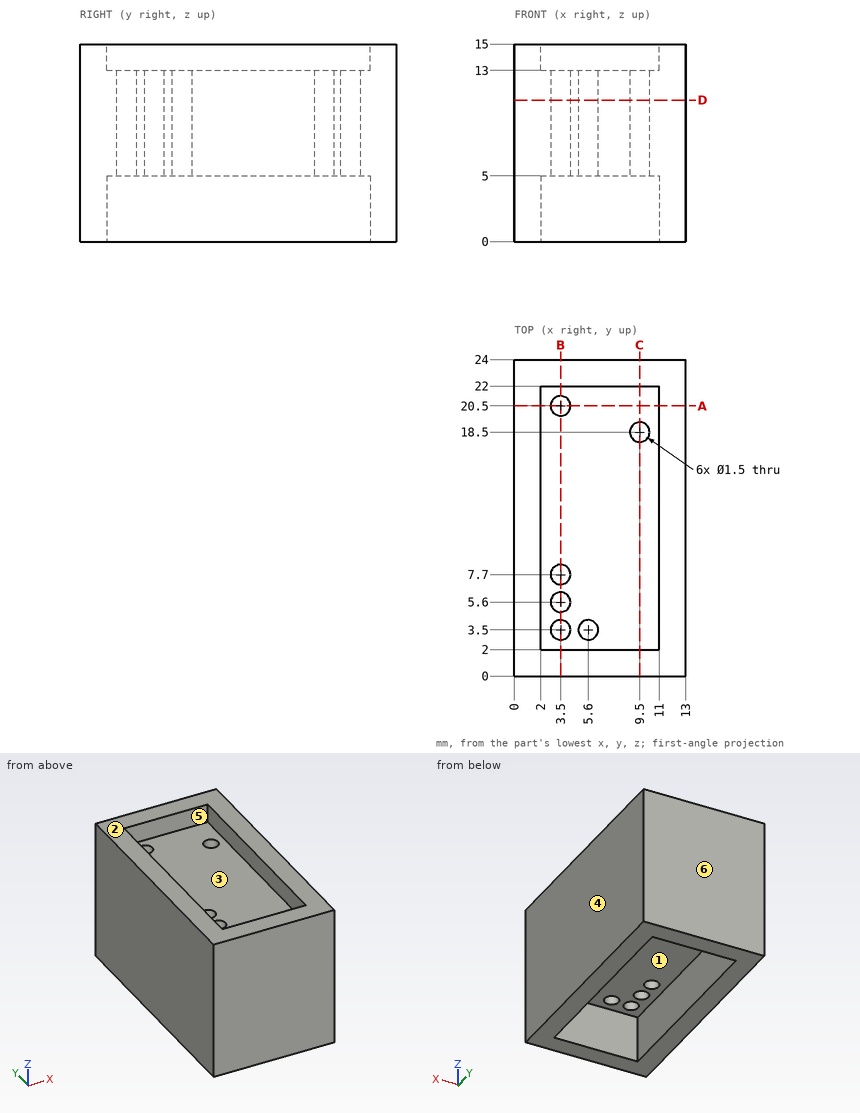
The drawing under review shows one solid part. Ordinate dimensions are in mm from its lowest x, y, z. A direction names the side the tool comes from. Give positions to 0.01 mm unless a question says otherwise; leave off trailing zeros. Write each loop counter-clockwise with the first axis right and the second up, starting at its lowest first coordinate (ties: lowest second). Pieces come first, ordered by that corner, then holes. Notation, with made-up numbers: (2, 20.5) -> (34, 20.5) arc R37 ccw to (34, 58.5) -> close; hole circle Ø10 at (38.5, 50). An arc over 180 degrees is marked (long way). Use CSV: the item, a comma, the result in double quotes.
Q1. To check wall thickness, follow probe 1 along Y at (x, z) = (3.5, 8.5); probe 2 along Y at (x, z) = (10.5, 4); probe 3 along Y at (x, z) = (5.6, 7.5). State the ranges of each line that lie inside material, in increasing order. Write a range as [from, to].
Conclusion:
probe 1,"[0, 2.75], [4.25, 4.85], [6.35, 6.95], [8.45, 19.75], [21.25, 24]"
probe 2,"[0, 2], [22, 24]"
probe 3,"[0, 2.75], [4.25, 24]"
Q2. Take a section at A-A, the plane y = 20.5. Write out the cut boundary in (x, z), then the cut area to 3 significant figures.
Conclusion:
outline,"(0, 0) -> (2, 0) -> (2, 5) -> (2.75, 5) -> (2.75, 13) -> (2, 13) -> (2, 15) -> (0, 15) -> close; (4.25, 5) -> (11, 5) -> (11, 0) -> (13, 0) -> (13, 15) -> (11, 15) -> (11, 13) -> (4.25, 13) -> close"
area,"120 mm2"
Q3. Take a section at B-B, the plane x = 3.5. Write out the cut boundary in (y, z), then the cut area to 3 significant figures.
Conclusion:
outline,"(0, 0) -> (2, 0) -> (2, 5) -> (2.75, 5) -> (2.75, 13) -> (2, 13) -> (2, 15) -> (0, 15) -> close; (4.25, 5) -> (4.85, 5) -> (4.85, 13) -> (4.25, 13) -> close; (6.35, 5) -> (6.95, 5) -> (6.95, 13) -> (6.35, 13) -> close; (8.45, 5) -> (19.75, 5) -> (19.75, 13) -> (8.45, 13) -> close; (21.25, 5) -> (22, 5) -> (22, 0) -> (24, 0) -> (24, 15) -> (22, 15) -> (22, 13) -> (21.25, 13) -> close"
area,"172 mm2"
Q4. Take a section at D-D, the plane z = 10.75. Write out the cut boundary in (x, y), then the cut area to 3 significant figures.
Conclusion:
outline,"(0, 0) -> (13, 0) -> (13, 24) -> (0, 24) -> close; hole circle Ø1.5 at (3.5, 3.5); hole circle Ø1.5 at (3.5, 5.6); hole circle Ø1.5 at (3.5, 7.7); hole circle Ø1.5 at (3.5, 20.5); hole circle Ø1.5 at (5.6, 3.5); hole circle Ø1.5 at (9.5, 18.5)"
area,"301 mm2"
Q5. Tool access review of the marked faces 1, 2 and 3: name each direction out of +Z, -Z, +X, -X, +Y, -Y from which nothing blocks a thin tool from reaching the whole face with its end or side.
Conclusion:
face 1,"-Z"
face 2,"+Z, +X, -X, +Y, -Y"
face 3,"+Z"
Q6. Take a section at C-C, the plane x = 9.5. Write out the cut boundary in (y, z), then the cut area to 3 significant figures.
Conclusion:
outline,"(0, 0) -> (2, 0) -> (2, 5) -> (17.75, 5) -> (17.75, 13) -> (2, 13) -> (2, 15) -> (0, 15) -> close; (19.25, 5) -> (22, 5) -> (22, 0) -> (24, 0) -> (24, 15) -> (22, 15) -> (22, 13) -> (19.25, 13) -> close"
area,"208 mm2"
Q7. For P1, Ø0.9, axis at x = 3.5, y = 3.5, coming from the -Z side; P2, Ø2, axis at x = 9.5, y = 18.5, coming from the -Z side; P3, Ø2.5, axis at x = 3.5, y = 20.5, coming from the +Z side, all flat-tipped, find the tip position at first contact; note any pin that passes through.
Conclusion:
P1,"through"
P2,"z = 5"
P3,"z = 13"
Q8. Mouldability with a two-part tool opening along Y and no side actions: class the marked faces 4, 5 and 6 as pulls with the +Y half, pulls with the -Y half, needs draft (parallel to the pull), parting line crosses it, or undercut.
Conclusion:
face 4,"needs draft"
face 5,"undercut"
face 6,"pulls with the +Y half"
